from build123d import *

# Parameters (mm, degrees)
SKETCH1_W           = 33
SKETCH1_H           = 33
BOSS_EXTRUDE1_DEPTH = 38
SKETCH2_R           = 8
BOSS_EXTRUDE2_DEPTH = 3
SKETCH3_R           = 3
BOSS_EXTRUDE3_DEPTH = 34
SKETCH4_W           = 4.9
SKETCH4_H           = 4.836057971
CUT_EXTRUDE1_DEPTH  = 17


with BuildPart() as part:
    # Sketch1 → Boss-Extrude1 (new body, symmetric)
    with BuildSketch(Plane(origin=(0, 0, 0), x_dir=(0, 0, -1), z_dir=(1, 0, 0))):
        Rectangle(SKETCH1_W, SKETCH1_H)
    extrude(amount=BOSS_EXTRUDE1_DEPTH, both=True)

    # Sketch2 → Boss-Extrude2 (add)
    with BuildSketch(Plane(origin=(38, 0, 0), x_dir=(0, 0, -1), z_dir=(1, 0, 0))):
        Circle(SKETCH2_R)
    extrude(amount=BOSS_EXTRUDE2_DEPTH)

    # Sketch3 → Boss-Extrude3 (add)
    with BuildSketch(Plane(origin=(41, 0, 0), x_dir=(0, 0, -1), z_dir=(1, 0, 0))):
        Circle(SKETCH3_R)
    extrude(amount=BOSS_EXTRUDE3_DEPTH)

    # Sketch4 → Cut-Extrude1 (cut, symmetric)
    with BuildSketch(Plane.XY):
        with Locations((52.55, 4.620557789)):
            Rectangle(SKETCH4_W, SKETCH4_H)
    extrude(amount=CUT_EXTRUDE1_DEPTH, both=True, mode=Mode.SUBTRACT)


solid = part.part
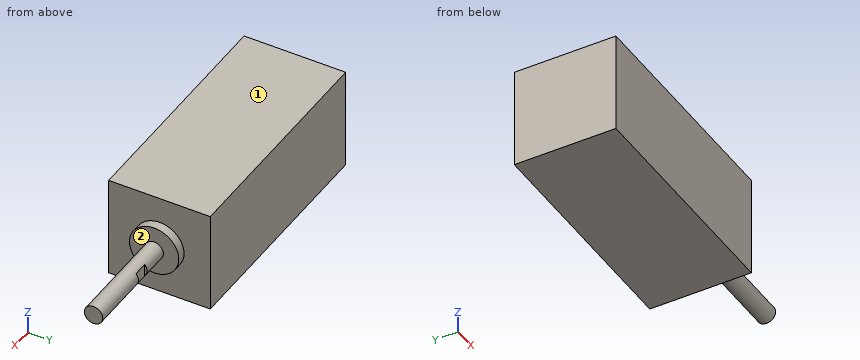
Source: CAD feature listing. Evaluate the final solid. Frame: model axes, mm. Face numbers are marked on the shaded views. A direction names the side the tool comes from. Coordinates: 2 decimals unless noted, no trailing zeros. Loops run counter-clockwise (first coordinate to the right, second up) from the corner with the lowest first, then second, coordinate; pieces in that order, holes last. Notation, with made-up numbers: M 0.25,-20 L 27.25,-20 A25 ccw 27.25,-6 Z; hole C 19.25,79 d3. An arc over 180 degrees is marked long. Answer in a Markdown table with one row per item.
Q1. Section A-A on z = 0. Return the cut outline in (x, y).
Answers below:
| item | result |
|---|---|
| outline | M -38,-16.5 L 38,-16.5 L 38,-8 L 41,-8 L 41,-3 L 75,-3 L 75,3 L 55,3 L 55,2.2 L 50.1,2.2 L 50.1,3 L 41,3 L 41,8 L 38,8 L 38,16.5 L -38,16.5 Z |
Q2. Section C-C on x = 63. Return the cut outline in (y, z).
Answers below:
| item | result |
|---|---|
| outline | C 0,0 d6 |
Q3. Section B-B on y = 0. Return the cut outline in (x, z).
Answers below:
| item | result |
|---|---|
| outline | M -38,-16.5 L 38,-16.5 L 38,-8 L 41,-8 L 41,-3 L 75,-3 L 75,3 L 41,3 L 41,8 L 38,8 L 38,16.5 L -38,16.5 Z |
Q4. Section D-D on y = -9. Return the cut outline in (x, z), plus the area to 3 significant figures.
Answers below:
| item | result |
|---|---|
| outline | M -38,-16.5 L 38,-16.5 L 38,16.5 L -38,16.5 Z |
| area | 2,510 mm^2 |
Q5. Ray query, probe 1 along X at (y, z) = (2.5, 1); probe 2 along X at (y, z) = (-9.5, -1.5); probe 3 along X at (y, z) = (5, 1). Return the intervals inside material, ascending. Write a range as from..to.
Answers below:
| item | result |
|---|---|
| probe 1 | x = -38..50.1, 55..75 |
| probe 2 | x = -38..38 |
| probe 3 | x = -38..41 |
Q6. Set-up query: the marked faces 1 and 2. Return all of +Z, -Z, +X, -X, +Y, -Y with unobstructed straight access to the full face (end or side cutting, diameter ignored); none if empty.
Answers below:
| item | result |
|---|---|
| face 1 | +Z, +X, -X, +Y, -Y |
| face 2 | +X |
Q7. First-contact query: pin 1 (5 mm diameter, centred on y = -3, z = 1, fed in from +X); pin 2 (10 mm diameter, centred on y = 9.5, z = 1.5, fed in from +X); pin 3 (3.5 mm diameter, centred on x = 52.5, z = -0.5, fed in from +Y); pin 4 (10 mm diameter, centred on y = -10, z = -11.5, fed in from +X). Flat tips, straight axial feed; report the tip coordinate or a pass-through.
Answers below:
| item | result |
|---|---|
| pin 1 | stops at x = 75 |
| pin 2 | stops at x = 41 |
| pin 3 | stops at y = 2.2 |
| pin 4 | stops at x = 38 |
